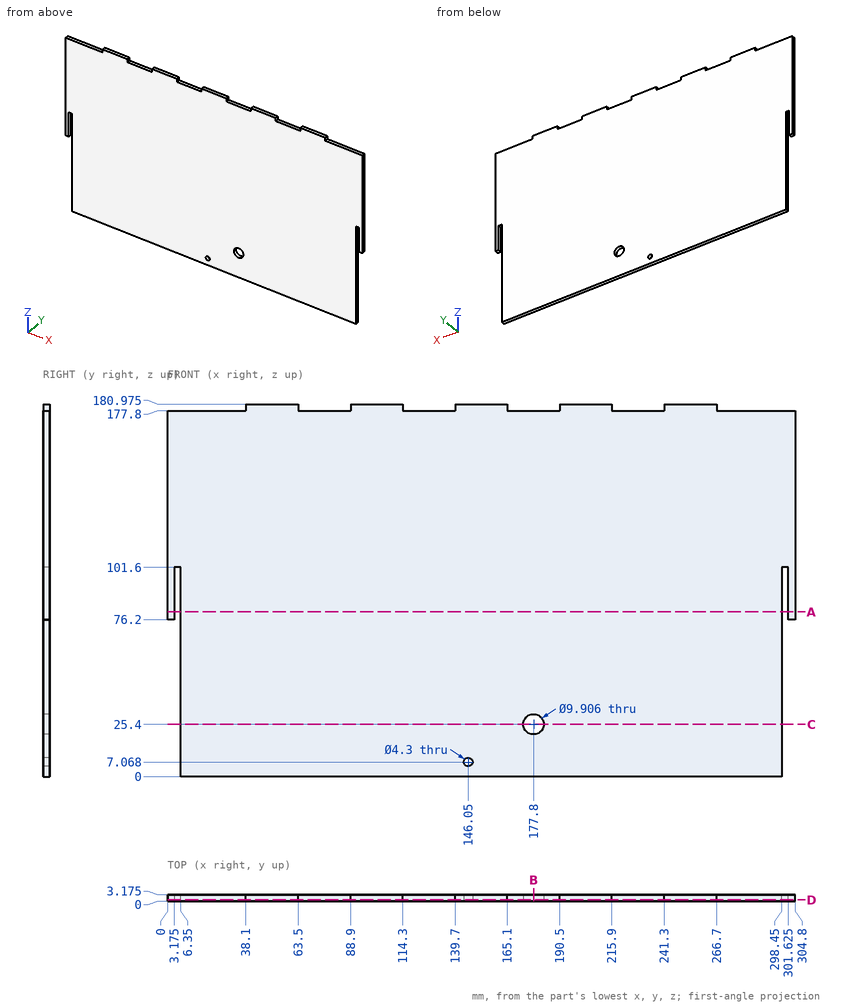
Job drawing, mm, ordinate dimensions from the low corner. One solid piece. Give positions to 0.01 mm unless a question says otherwise; leave off trailing zeros. Write each loop counter-clockwise with the first axis right and the second up, starting at its lowest first coordinate (ties: lowest second). Pieces come first, ordered by that corner, then holes. Notation, with made-up numbers: (24.5, 45.25) -> (47.5, 45.25) arc R36 ccw to (47.5, 81.25) -> close; hole circle Ø6 at (2, 38.25). An arc over 180 degrees is marked (long way). Return JSON: item names as keys, results as strings.
Item 1: Band-saw the part on A-A (z = 80). List the corners of the cut face in (x, y) (3 decimals).
Answer below:
{"outline": "(0, 0) -> (3.175, 0) -> (3.175, 3.175) -> (0, 3.175) -> close; (6.35, 0) -> (298.45, 0) -> (298.45, 3.175) -> (6.35, 3.175) -> close; (301.625, 0) -> (304.8, 0) -> (304.8, 3.175) -> (301.625, 3.175) -> close"}
Item 2: Band-saw the part on D-D (y = 0.65). Give the number of separate pieces and of enclosed holes in the cut face, then the cut area to 3 significant figures.
Answer below:
{"separate pieces": "1", "enclosed holes": "2", "area": "53,400 mm2"}
Item 3: Band-saw the part on C-C (z = 25.4). List the corners of the cut face in (x, y) (3 decimals).
Answer below:
{"outline": "(6.35, 0) -> (172.847, 0) -> (172.847, 3.175) -> (6.35, 3.175) -> close; (182.753, 0) -> (298.45, 0) -> (298.45, 3.175) -> (182.753, 3.175) -> close"}
Item 4: Band-saw the part on B-B (x = 177.8). List the corners of the cut face in (y, z) (3 decimals), then the cut area to 3 significant figures.
Answer below:
{"outline": "(0, 0) -> (3.175, 0) -> (3.175, 20.447) -> (0, 20.447) -> close; (0, 30.353) -> (3.175, 30.353) -> (3.175, 177.8) -> (0, 177.8) -> close", "area": "533 mm2"}
Item 5: Drill centre lines: probe 1 along Z at (x, y) = (146.05, 1.75) (1 decimal); probe 2 along X at (y, z) = (2, 80.5) (3 decimals); probe 3 along Z at (x, y) = (136.5, 2). Where is each one in solid material? Low to high.
Answer below:
{"probe 1": "z = 0 to 4.9, 9.2 to 181", "probe 2": "x = 0 to 3.175, 6.35 to 298.45, 301.625 to 304.8", "probe 3": "z = 0 to 177.8"}
Item 6: Drop flat-ended pins along their axis: pin 1 (1.6 mm diameter, centred on x = 17.5, y = 1, fed in from +Z); pin 2 (1.6 mm diameter, centred on y = 1.5, z = 179, fed in from +X); pin 3 (1 mm diameter, centred on x = 300, y = 1, fed in from -Z); pin 4 (1 mm diameter, centred on y = 2.5, z = 113, fed in from -X). Give the stop position or say it passes through.
Answer below:
{"pin 1": "stops at z = 177.8", "pin 2": "stops at x = 266.7", "pin 3": "stops at z = 101.6", "pin 4": "stops at x = 0"}
